Can you work these out from the model? Positions are in its coordinate system, mm. Face numbers are marked on the shaded views. A direction names the side the tool comes from. Round coordinates to 2 decimals unless told otherwise and drop trailing zeros. Loops run counter-clockwise (first coordinate to the right, second up) from the corner with the lowest first, then second, coordinate; pieces in that order, holes last.
(1) I want a section at C-C on x = 54.5. Write out the boundary of the cut face in (y, z).
(2) If I drill on line 1 along X through (y, z) = (19, -6); line 2 along Y through (x, z) = (44.5, 1); line 3 along Z through (x, y) = (23, 0.5), over which ranges is the centre line in solid material (lowest first)?
(3) I want a section at D-D on x = 43.5. Write out the boundary of the cut face in (y, z).
(4) I want a section at B-B on y = 0. Write out the boundary of the cut face in (x, z), plus the area to 3 significant figures.
(5) I want a section at A-A on z = 0. Write out the boundary of the cut face in (x, y), plus the area to 3 significant figures.
(6) Will these pins go through, and if not, where does the flat tip stop? pin 1 Ø2 at (x, z) = (38.5, 1.5) entering from +Y; pin 2 Ø8 at (x, z) = (53.5, 8.5) entering from +Y; pin 3 Ø10 at (x, z) = (42, -6.5) entering from +Y; pin 4 Ø1 at (y, z) = (1, -16) entering from -X.
(7) Which directions (+Z, -Z, +X, -X, +Y, -Y) give clear straight access to the entire face, cutting with the end or side of a thin tool? Please do the marked faces 1 and 2.
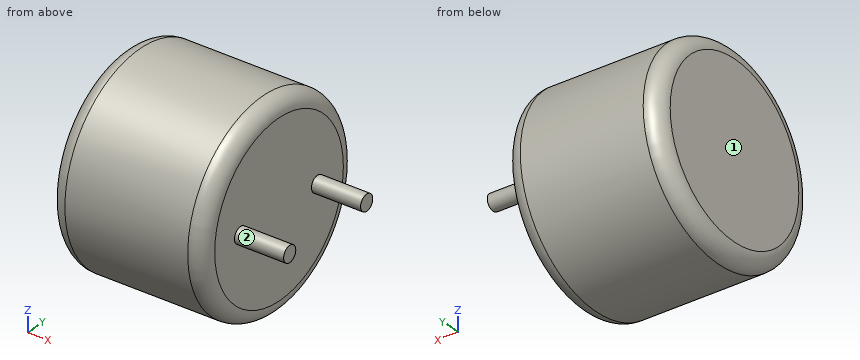
from build123d import *

# Parameters (mm, degrees)
F0_R     = 32.5735
F1_DEPTH = 50
F2_R     = 5
F3_R     = 2.6
F4_DEPTH = 16


with BuildPart() as f1:
    # F0 (on Right) → F1 (new body)
    with BuildSketch(Plane.YZ):
        Circle(F0_R)
    extrude(amount=F1_DEPTH)

    # F2
    f2_edges = [f1.edges().sort_by_distance(p)[0] for p in [
        (50, -32.5735, 0),
        (0, -32.5735, 0),
    ]]
    fillet(f2_edges, radius=F2_R)

    # F3 (on face) → F4 (join)
    with BuildSketch(Plane.YZ.offset(50)):
        with Locations((16.5, 0)):
            Circle(F3_R)
        with Locations((-16.5, 0)):
            Circle(F3_R)
    extrude(amount=F4_DEPTH)


solid = f1.part
Filled sheet:
1. outline: circle Ø5.2 at (-16.5, 0); circle Ø5.2 at (16.5, 0)
2. line 1: x = 0 to 50
2. line 2: y = -32.56 to 32.56
2. line 3: z = -32.57 to 32.57
3. outline: circle Ø65.15 at (0, 0)
4. outline: (0, -27.57) arc R5 ccw to (5, -32.57) - (45, -32.57) arc R5 ccw to (50, -27.57) - (50, 27.57) arc R5 ccw to (45, 32.57) - (5, 32.57) arc R5 ccw to (0, 27.57) - close
4. area: 3,240 mm2
5. outline: (0, -27.57) arc R5 ccw to (5, -32.57) - (45, -32.57) arc R5 ccw to (50, -27.57) - (50, -19.1) - (66, -19.1) - (66, -13.9) - (50, -13.9) - (50, 13.9) - (66, 13.9) - (66, 19.1) - (50, 19.1) - (50, 27.57) arc R5 ccw to (45, 32.57) - (5, 32.57) arc R5 ccw to (0, 27.57) - close
5. area: 3,400 mm2
6. pin 1: stops at y = 32.57
6. pin 2: stops at y = 28.59
6. pin 3: stops at y = 32.54
6. pin 4: stops at x = 0
7. face 1: +Z, -Z, -X, +Y, -Y
7. face 2: +X
